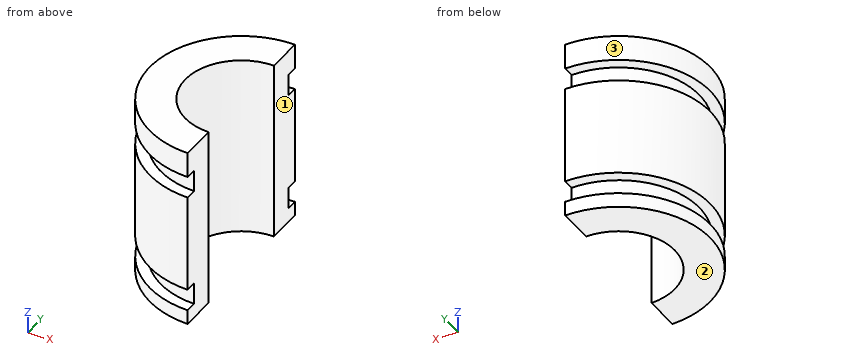
from build123d import *

# Parameters (mm, degrees)
Y_KSEKLIK_EKSTR_ZYON1_DEPTH = 25
IZIM2_W                     = 3
IZIM2_H                     = 1.5


with BuildPart() as part:
    # Çizim1 → Yükseklik-Ekstrüzyon1 (new body)
    with BuildSketch(Plane.XY):
        with BuildLine():
            Line((0, 12.5), (0, 7.65))
            ThreePointArc((0, 7.65), (-7.65, 0), (0, -7.65))
            Line((0, -7.65), (0, -12.5))
            ThreePointArc((0, -12.5), (-12.5, 0), (0, 12.5))
        make_face()
    extrude(amount=Y_KSEKLIK_EKSTR_ZYON1_DEPTH)

    # Çizim2 → Kes-Döndür1 (revolve, cut)
    with BuildSketch(Plane(origin=(0, 0, 0), x_dir=(0, 0, -1), z_dir=(1, 0, 0))):
        with Locations((-20, 11.75)):
            Rectangle(IZIM2_W, IZIM2_H)
        with Locations((-3.5, 11.75)):
            Rectangle(IZIM2_W, IZIM2_H)
    revolve(axis=Axis((0, 0, 0), (0, 0, 1)), mode=Mode.SUBTRACT)


solid = part.part
Model file for the job. Use its own axes, mm. Face numbers are marked on the shaded views. Round coordinates to 2 decimals unless told otherwise and drop trailing zeros. Order: outer loops, then holes, each group sorted by start corner. A loop starts at its lowest first (then second) coordinate and runs counter-clockwise, first axis right, second up.
(1) Pull direction X, two halves, no side cores. Call the marked faces 1, 2 and 3: released by +X, released by -X, zero draft, split by the parting line, or undercut.
(2) Pin check, flat tips, straight feed: pin 1 (2 mm diameter, centred on y = -7, z = 11, fed in from -X); pin 2 (5 mm diameter, centred on x = -6.5, z = 16.5, fed in from +Y); pin 3 (1.5 mm diameter, centred on y = 5, z = 11, fed in from -X). Stop position of each tip, or through.
(3) Band-saw the part on C-C (z = 8.25). List the corners of the cut face in (x, y), then the cut area to 3 significant figures.
(4) Band-saw the part on A-A (x = -4). List the corners of the cut face in (y, z).
(5) Drill centre lines: line 1 (Z direction, x = -1.5, y = 11.75); line 2 (X direction, y = 0, z = 2.75); line 3 (Y direction, x = -5.5, z = 3.25). Where is each one in solid material? Low to high.
(6) Band-saw the part on D-D (x = -9.75). List the corners of the cut face in (y, z).
(7) Band-saw the part on B-B (y = 8.75). List the corners of the cut face in (x, z), then the cut area to 3 significant figures.
Verdict:
1. face 1: released by +X
1. face 2: zero draft
1. face 3: released by -X
2. pin 1: stops at x = -10.97
2. pin 2: stops at y = 11.84
2. pin 3: stops at x = -11.76
3. outline: (0, -12.5) - (0, -7.65) arc R7.65 cw to (0, 7.65) - (0, 12.5) arc R12.5 ccw to start
3. area: 154 mm2
4. outline: (-11.84, 0) - (-6.52, 0) - (-6.52, 25) - (-11.84, 25) - (-11.84, 21.5) - (-10.25, 21.5) - (-10.25, 18.5) - (-11.84, 18.5) - (-11.84, 5) - (-10.25, 5) - (-10.25, 2) - (-11.84, 2) - close; (6.52, 0) - (11.84, 0) - (11.84, 2) - (10.25, 2) - (10.25, 5) - (11.84, 5) - (11.84, 18.5) - (10.25, 18.5) - (10.25, 21.5) - (11.84, 21.5) - (11.84, 25) - (6.52, 25) - close
5. line 1: z = 0 to 2, 5 to 18.5, 21.5 to 25
5. line 2: x = -11 to -7.65
5. line 3: y = -9.53 to -5.32, 5.32 to 9.53
6. outline: (-7.82, 0) - (7.82, 0) - (7.82, 2) - (5.09, 2) - (5.09, 5) - (7.82, 5) - (7.82, 18.5) - (5.09, 18.5) - (5.09, 21.5) - (7.82, 21.5) - (7.82, 25) - (-7.82, 25) - (-7.82, 21.5) - (-5.09, 21.5) - (-5.09, 18.5) - (-7.82, 18.5) - (-7.82, 5) - (-5.09, 5) - (-5.09, 2) - (-7.82, 2) - close
7. outline: (-8.93, 0) - (0, 0) - (0, 25) - (-8.93, 25) - (-8.93, 21.5) - (-6.67, 21.5) - (-6.67, 18.5) - (-8.93, 18.5) - (-8.93, 5) - (-6.67, 5) - (-6.67, 2) - (-8.93, 2) - close
7. area: 210 mm2
